```python
from build123d import *

# Parameters (mm, degrees)
SKETCH1_W            = 127.7
SKETCH1_H            = 85.9
BOSS_EXTRUDE1_DEPTH  = 15
SKETCH2_R            = 6
CUT_EXTRUDE1_DEPTH   = 12
LPATTERN3_COUNT      = 8
LPATTERN3_PITCH      = 15
LPATTERN3_COUNT_DIR2 = 5
LPATTERN3_PITCH_DIR2 = 14
SKETCH3_R            = 2
CUT_EXTRUDE2_DEPTH   = 12
LPATTERN4_COUNT      = 8
LPATTERN4_PITCH      = 15
LPATTERN4_COUNT_DIR2 = 5
LPATTERN4_PITCH_DIR2 = 14


with BuildPart() as part:
    # Sketch1 → Boss-Extrude1 (new body)
    with BuildSketch(Plane(origin=(0, 0, 0), x_dir=(1, 0, 0), z_dir=(0, 1, 0))):
        with Locations((-248.856003869, 89.066665881)):
            Rectangle(SKETCH1_W, SKETCH1_H)
    extrude(amount=BOSS_EXTRUDE1_DEPTH)

    # Sketch2 → Cut-Extrude1 (cut)
    with BuildSketch(Plane(origin=(0, 15, 0), x_dir=(1, 0, 0), z_dir=(0, 1, 0))):
        with Locations((-302.706003869, 112.016665881)):
            Circle(SKETCH2_R)
    cut_extrude1 = extrude(amount=-CUT_EXTRUDE1_DEPTH, mode=Mode.SUBTRACT)

    # LPattern3: Cut-Extrude1 8 × 5
    with Locations(*[(i * LPATTERN3_PITCH, 0, j * LPATTERN3_PITCH_DIR2) for i in range(LPATTERN3_COUNT) for j in range(LPATTERN3_COUNT_DIR2) if (i, j) != (0, 0)]):
        add(cut_extrude1, mode=Mode.SUBTRACT)

    # Sketch3 → Cut-Extrude2 (cut)
    with BuildSketch(Plane(origin=(0, 3, 0), x_dir=(1, 0, 0), z_dir=(0, 1, 0))):
        with Locations((-302.706003869, 112.016665881)):
            Circle(SKETCH3_R)
    cut_extrude2 = extrude(amount=-CUT_EXTRUDE2_DEPTH, mode=Mode.SUBTRACT)

    # LPattern4: Cut-Extrude2 8 × 5
    with Locations(*[(i * LPATTERN4_PITCH, 0, j * LPATTERN4_PITCH_DIR2) for i in range(LPATTERN4_COUNT) for j in range(LPATTERN4_COUNT_DIR2) if (i, j) != (0, 0)]):
        add(cut_extrude2, mode=Mode.SUBTRACT)


solid = part.part
```
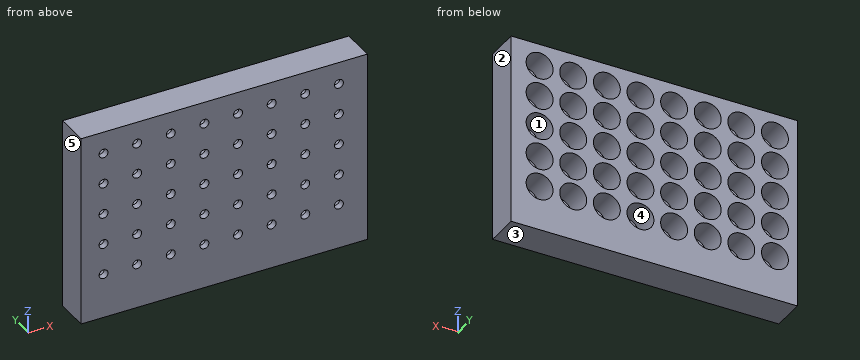
The listing builds one solid part. Answer for the finished solid, in the listing's coordinates (mm). Face numbers are marked on the shaded views. A direction names the side the tool comes from. Coordinates: 2 decimals unless noted, no trailing zeros. Loops run counter-clockwise (first coordinate to the right, second up) from the corner with the lowest first, then second, coordinate; pieces in that order, holes last. Notation, with made-up numbers: (3, -20) -> (26, -20) arc R38 ccw to (26, 18) -> close; hole circle Ø5 at (-7.5, 77.5). An arc over 180 degrees is marked (long way). Return JSON: item names as keys, results as strings. Group by question number.
(1) Which of the six approach directions +Z, -Z, +X, -X, +Y, -Y give full straight-line access (tool end or side, diameter ignored) to the marked faces 1 and 2?
(2) Find the intervals of material crossed by probe 1 along Z at (x, y) = (-214.5, 8.5); probe 2 along Z at (x, y) = (-298.5, 6); probe 3 along Y at (x, z) = (-297.5, -56), in increasing order. Write a range as from..to.
(3) A cutting plane is placed at C-C on x = -254. Write down the section's boundary in (y, z), and give its area (3 significant figures).
(4) A cutting plane is placed at A-A on x = -208.5. Write down the section's boundary in (y, z).
(5) Given pin 1 Ø7 at (x, z) = (-227.71, -84.02) entering from +Y, flat-ended and moving along its own axis, determine where the tip first touches the part or whether it passes through.
(6) A cutting plane is placed at B-B on y = 11.5. Count the separate pieces of the cut face and the enclosed holes in it, and give its area (3 significant figures).
(7) Determine the mould class of the marked faces 3, 4 and 5 for opening direction Z: released by +Z, released by -Z, zero draft, split by the parting line, or undercut.
The answers:
{
 "1": {"face 1": "+Y", "face 2": "+Z, -Z, +X, +Y, -Y"},
 "2": {"probe 1": "z = -132.02..-117.74, -106.29..-103.74, -92.29..-89.74, -78.29..-75.74, -64.29..-61.74, -50.29..-46.12", "probe 2": "z = -132.02..-116.3, -107.74..-102.3, -93.74..-88.3, -79.74..-74.3, -65.74..-60.3, -51.74..-46.12", "probe 3": "y = 0..3"},
 "3": {"outline": "(0, -132.02) -> (15, -132.02) -> (15, -116.74) -> (3, -116.74) -> (3, -107.3) -> (15, -107.3) -> (15, -102.74) -> (3, -102.74) -> (3, -93.3) -> (15, -93.3) -> (15, -88.74) -> (3, -88.74) -> (3, -79.3) -> (15, -79.3) -> (15, -74.74) -> (3, -74.74) -> (3, -65.3) -> (15, -65.3) -> (15, -60.74) -> (3, -60.74) -> (3, -51.3) -> (15, -51.3) -> (15, -46.12) -> (0, -46.12) -> close", "area": "722 mm^2"},
 "4": {"outline": "(0, -132.02) -> (15, -132.02) -> (15, -116.3) -> (3, -116.3) -> (3, -107.74) -> (15, -107.74) -> (15, -102.3) -> (3, -102.3) -> (3, -93.74) -> (15, -93.74) -> (15, -88.3) -> (3, -88.3) -> (3, -79.74) -> (15, -79.74) -> (15, -74.3) -> (3, -74.3) -> (3, -65.74) -> (15, -65.74) -> (15, -60.3) -> (3, -60.3) -> (3, -51.74) -> (15, -51.74) -> (15, -46.12) -> (0, -46.12) -> close"},
 "5": {"pin 1": "stops at y = 3"},
 "6": {"separate pieces": "1", "enclosed holes": "40", "area": "6,450 mm^2"},
 "7": {"face 3": "released by -Z", "face 4": "undercut", "face 5": "zero draft"}
}
